For this review, use the dimensioned drawing (mm, ordinates from the lowest corner) and the shaded views. A direction names the side the tool comes from. Coordinates: 2 decimals unless noted, no trailing zeros. Loops run counter-clockwise (first coordinate to the right, second up) from the corner with the lowest first, then second, coordinate; pieces in that order, holes last. Notation, with made-up numbers: (-26, 52) -> (26, 52) arc R22 ccw to (26, 86) -> close; hole circle Ø1 at (-28, 23.5). An arc over 180 degrees is marked (long way). Answer as a JSON object with one key per item and string values.
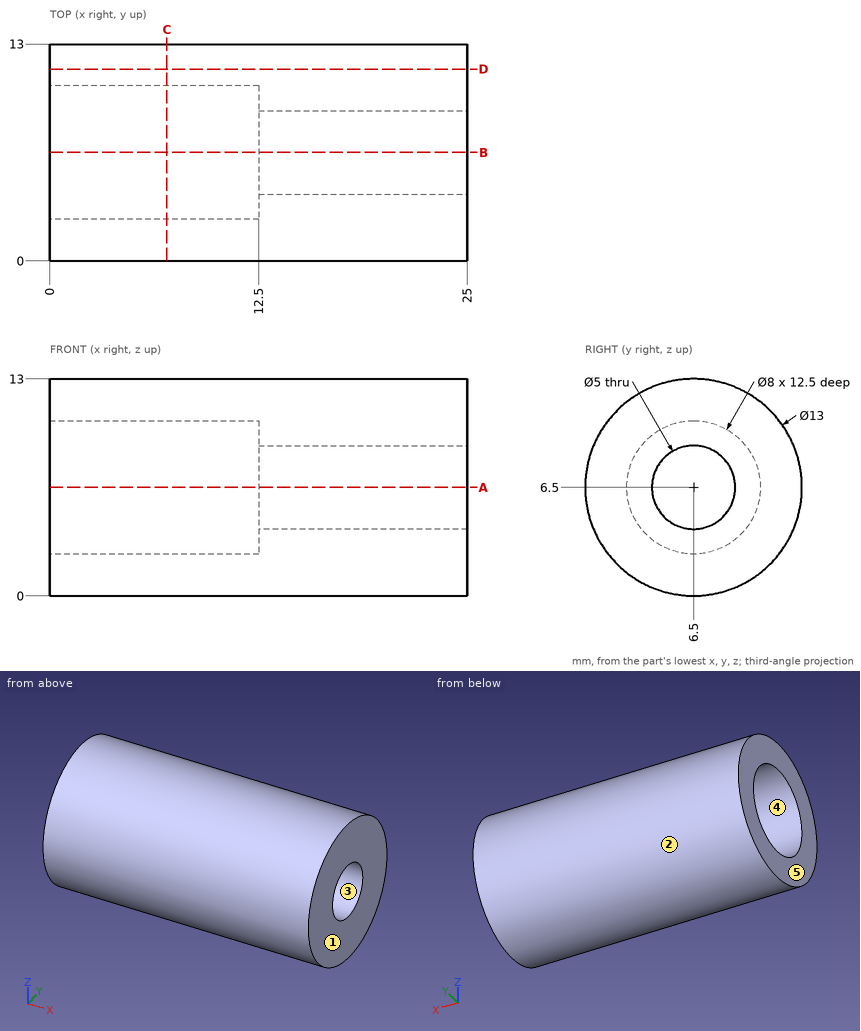
1) Clearance check with flat-ended pins moving along their axes: pin 1 Ø3 at (x, y) = (6.5, 10) entering from +Z; pin 2 Ø2.5 at (y, z) = (6.5, 5.5) entering from -X (3 decimals); pin 3 Ø6 at (x, z) = (20, 5) entering from -Y; pin 4 Ø6 at (x, z) = (7, 11) entering from +Y. State where each tip first meets the part, or that it passes through.
Completed:
{"pin 1": "z = 12.68", "pin 2": "through", "pin 3": "y = 0", "pin 4": "y = 12.82"}
2) For the marked faces 4 and 5, list the 3-axis set-ups (+Z, -Z, +X, -X, +Y, -Y) from which the entire face can be reached by the end or side of a thin tool; tool diameter is ignored.
Completed:
{"face 4": "-X", "face 5": "+Z, -Z, -X, +Y, -Y"}
3) Wall thickness on probe 1 along Y at (x, z) = (7.75, 6.5); probe 2 along Y at (x, z) = (20.5, 6.5); probe 3 along Z at (x, y) = (21.25, 7.5): over which ranges is each line inside the solid? List them lowest first.
Completed:
{"probe 1": "0 to 2.5, 10.5 to 13", "probe 2": "0 to 4, 9 to 13", "probe 3": "0.08 to 4.21, 8.79 to 12.92"}
4) Add section D-D, the plane y = 11.5. Give the boundary of the cut face in (x, z), and give its area (3 significant figures).
Completed:
{"outline": "(0, 2.35) -> (25, 2.35) -> (25, 10.65) -> (0, 10.65) -> close", "area": "208 mm²"}
5) Add section A-A, the plane z = 6.5. Give the boundary of the cut face in (x, y), and give its area (4 significant figures).
Completed:
{"outline": "(0, 0) -> (25, 0) -> (25, 4) -> (12.5, 4) -> (12.5, 2.5) -> (0, 2.5) -> close; (0, 10.5) -> (12.5, 10.5) -> (12.5, 9) -> (25, 9) -> (25, 13) -> (0, 13) -> close", "area": "162.5 mm²"}
6) The part is to be moulded in two halves that separate along Z. For the marked faces 1, 2 and 3, say which applies: pulls with the +Z half, pulls with the -Z half, needs draft (parallel to the pull), parting line crosses it, or undercut.
Completed:
{"face 1": "needs draft", "face 2": "parting line crosses it", "face 3": "undercut"}
7) Add section C-C, the plane x = 7. Give the boundary of the cut face in (y, z).
Completed:
{"outline": "circle Ø13 at (6.5, 6.5); hole circle Ø8 at (6.5, 6.5)"}
